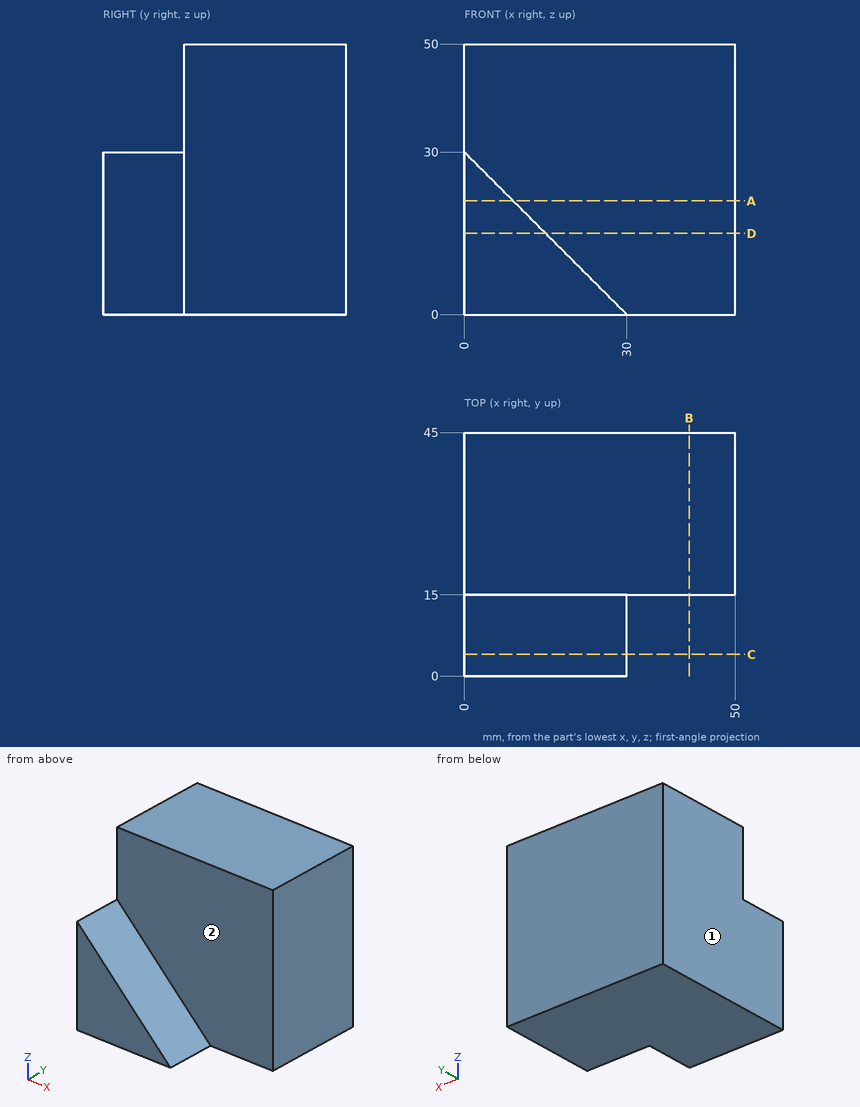
Could you check a few things on this drawing? It's one solid part, dimensions in mm from its lowest x, y, z. A direction names the side the tool comes from. Give positions to 0.01 mm unless a question says otherwise; leave off trailing zeros. Loops run counter-clockwise (first coordinate to the right, second up) from the corner with the lowest first, then second, coordinate; pieces in that order, holes last. Notation, with made-up numbers: M 3,7 L 45,7 A28 cw 45,30 Z; hole C 70.5,63 d11. An arc over 180 degrees is marked long. One line per question, with ' | ' between items. Start each with the question number.
Q1. If we section it at A-A (z = 21): Please give me the cut outline in (x, y), plus the area to 4 significant figures.
Q2. For pin 1 Ø6 at (x, z) = (29.5, 16) entering from -Y, with a flat end and sliding along its axis, tell me the tip position at first contact or that it passes through.
Q3. For the marked faces 1 and 2, which set-ups out of +Z, -Z, +X, -X, +Y, -Y let a thin tool reach every point of the face, with its end or its side?
Q4. If I drill on line 1 (Y direction, x = 21, z = 13.5); line 2 (Z direction, x = 20, y = 14); line 3 (Z direction, x = 7, y = 3.5), over which ranges is the centre line in solid material (lowest first)? Write a range as from..to.
Q5. If we section it at B-B (x = 41.5): Please give me the cut outline in (y, z).
Q6. If we section it at C-C (y = 4): Please give me the cut outline in (x, z), plus the area to 3 significant figures.
Q7. If we section it at D-D (z = 15): Please give me the cut outline in (x, y), plus the area to 4 significant figures.
Computed:
1) outline: M 0,0 L 9,0 L 9,15 L 50,15 L 50,45 L 0,45 Z | area: 1,635 mm²
2) pin 1: stops at y = 15
3) face 1: +Z, -Z, -X, +Y, -Y | face 2: +Z, +X, -Y
4) line 1: y = 15..45 | line 2: z = 0..10 | line 3: z = 0..23
5) outline: M 15,0 L 45,0 L 45,50 L 15,50 Z
6) outline: M 0,0 L 30,0 L 0,30 Z | area: 450 mm²
7) outline: M 0,0 L 15,0 L 15,15 L 50,15 L 50,45 L 0,45 Z | area: 1,725 mm²
